The listing builds one solid part. Answer for the finished solid, in the listing's coordinates (mm). Give positions to 0.01 mm unless a question says otherwise; leave off trailing zeros. Order: outer loops, then holes, each group sorted by start corner. A loop starts at its lowest first (then second) coordinate and runs counter-clockwise, first axis right, second up. Notation, with made-up numbers: (73.5, 56.25) - (128.5, 56.25) arc R16 cw to (128.5, 83.25) - close; hole circle Ø2 at (40.25, 78.5). An arc over 180 degrees is marked (long way). Use CSV: the item, a comma, the result in double quotes.
```python
from build123d import *

# Parameters (mm, degrees)
BOSS_EXTRUDE1_DEPTH = 3
SKETCH2_R           = 1.75
CUT_EXTRUDE1_DEPTH  = 4


with BuildPart() as part:
    # Sketch1 → Boss-Extrude1 (new body)
    with BuildSketch(Plane(origin=(0, 0, 0), x_dir=(0, 0, -1), z_dir=(1, 0, 0))):
        Polygon((0, 0), (0, 50), (34, 80), (154, 80), (154, 0), align=None)
    extrude(amount=BOSS_EXTRUDE1_DEPTH)

    # Sketch2 → Cut-Extrude1 (cut, through all)
    with BuildSketch(Plane.ZY):
        with Locations((-149, 5)):
            Circle(SKETCH2_R)
        with Locations((-149, 75)):
            Circle(SKETCH2_R)
        with Locations((-5, 5)):
            Circle(SKETCH2_R)
        with Locations((-55.407189005, 75)):
            Circle(SKETCH2_R)
        with Locations((-18.540830268, 51.422993608)):
            Circle(SKETCH2_R)
    extrude(amount=-CUT_EXTRUDE1_DEPTH, mode=Mode.SUBTRACT)


solid = part.part
```
Item 1: The part is cut by section D-D (y = 75). Give the vertices of the cut face in (x, z), and give its area (3 significant figures).
Taken from the geometry:
outline,"(0, -154) - (3, -154) - (3, -150.75) - (0, -150.75) - close; (0, -147.25) - (3, -147.25) - (3, -57.16) - (0, -57.16) - close; (0, -53.66) - (3, -53.66) - (3, -28.33) - (0, -28.33) - close"
area,"356 mm^2"
Item 2: The part is cut by section A-A (y = 5). Give the vertices of the cut face in (x, z), and give its area (3 significant figures).
Taken from the geometry:
outline,"(0, -154) - (3, -154) - (3, -150.75) - (0, -150.75) - close; (0, -147.25) - (3, -147.25) - (3, -6.75) - (0, -6.75) - close; (0, -3.25) - (3, -3.25) - (3, 0) - (0, 0) - close"
area,"441 mm^2"
Item 3: Find the intervals of material crossed by line 1 along Y through (x, z) = (1.3, -149); line 2 along Z through (x, y) = (1.35, 75); line 3 along Y through (x, z) = (1.5, -5), in increasing order.
Taken from the geometry:
line 1,"0 to 3.25, 6.75 to 73.25, 76.75 to 80"
line 2,"-154 to -150.75, -147.25 to -57.16, -53.66 to -28.33"
line 3,"0 to 3.25, 6.75 to 54.41"
Item 4: The part is cut by section C-C (z = -5). Give the vertices of the cut face in (x, y).
Taken from the geometry:
outline,"(0, 0) - (3, 0) - (3, 3.25) - (0, 3.25) - close; (0, 6.75) - (3, 6.75) - (3, 54.41) - (0, 54.41) - close"
Item 5: The mould has two halves that part along Z. Classify faces 1 (the face through (1, 41, -154)), 2 (the face through (1, 80, -93)), 3 (the face through (1, 25, 0)), 4 (the face through (1.48, 3.29, -5.38)): +Z half, -Z half, draft (parallel to the pull), parting line (faces both ways), or undercut.
Taken from the geometry:
face 1,"-Z half"
face 2,"draft"
face 3,"+Z half"
face 4,"undercut"
Item 6: The part is cut by section B-B (x = 0.45). Give the vertices of the cut face in (y, z).
Taken from the geometry:
outline,"(0, -154) - (80, -154) - (80, -34) - (50, 0) - (0, 0) - close; hole circle Ø3.5 at (5, -149); hole circle Ø3.5 at (5, -5); hole circle Ø3.5 at (51.42, -18.54); hole circle Ø3.5 at (75, -149); hole circle Ø3.5 at (75, -55.41)"
